Job drawing, mm, ordinate dimensions from the low corner. One solid piece. Give positions to 0.01 mm unless a question says otherwise; leave off trailing zeros. Order: outer loops, then holes, each group sorted by start corner. A loop starts at its lowest first (then second) coordinate and runs counter-clockwise, first axis right, second up.
Item 1: Flat gauge pins, fed straight in: P1, Ø1, axis at x = 21, y = 62.5, coming from the +Z side; P2, Ø12, axis at x = 24.5, z = 135.5, coming from the -Y side. Where does each tip first touch, or does it go through?
Item 2: Band-saw the part on D-D on x = 125. Give the cut face in (y, z), plus the area to 3 significant figures.
Item 3: Band-saw the part on A-A on x = 30. Give the cut face in (y, z), plus the area to 3 significant figures.
Item 4: Two-plate mould, pull along Z, no slides. Class the marked faces 1, 2 and 3: released by +Z, released by -Z, zero draft, split by the parting line, or undercut.
Item 5: Band-saw the part on C-C on y = 46. Give the cut face in (x, z), plus the area to 3 significant figures.
Item 6: Band-saw the part on B-B on z = 170. Give the cut face in (x, y).
Item 7: Wall check: L1, parallel to X at y = 125.5, z = 31; L2, parallel to Y at x = 93.5, z = 170.5; L3, parallel to Z at x = 23.5, y = 138.5. Give the ranges that are in metal, low to high.
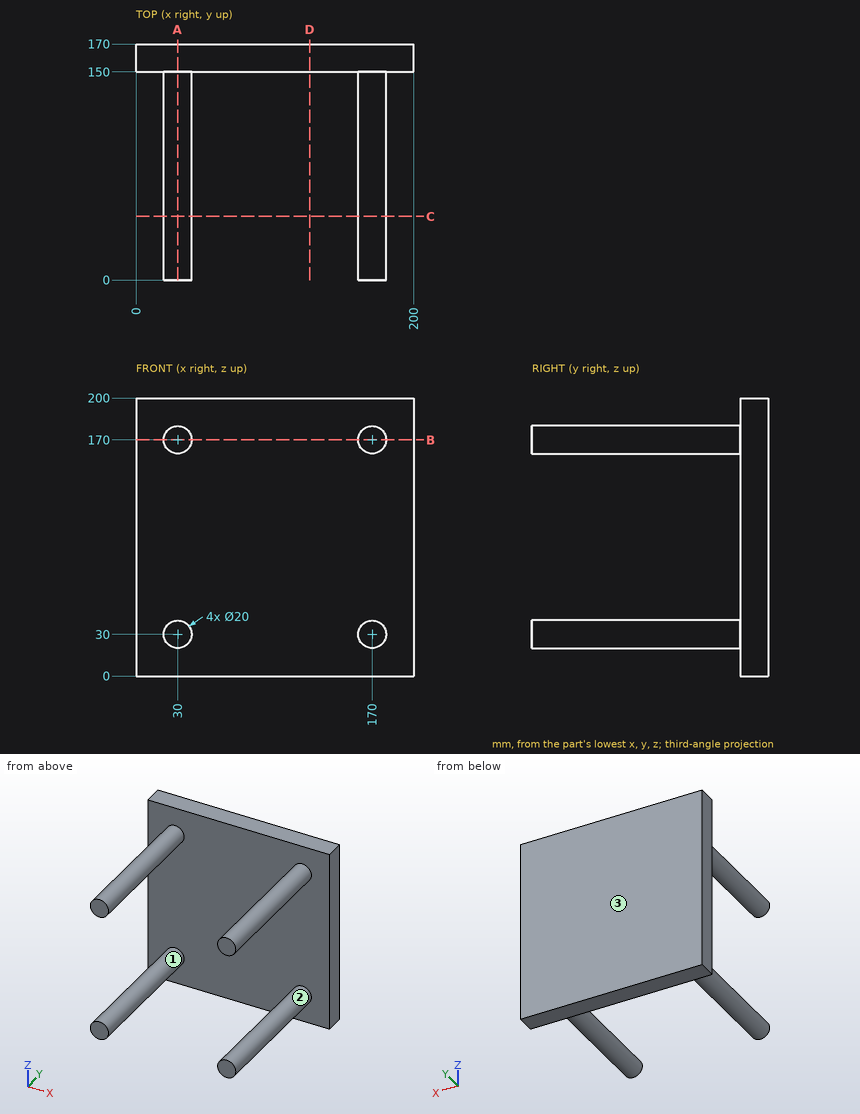
The answers:
1. P1: stops at z = 175.27
1. P2: stops at y = 150
2. outline: (150, 0) - (170, 0) - (170, 200) - (150, 200) - close
2. area: 4,000 mm2
3. outline: (0, 20) - (150, 20) - (150, 0) - (170, 0) - (170, 200) - (150, 200) - (150, 180) - (0, 180) - (0, 160) - (150, 160) - (150, 40) - (0, 40) - close
3. area: 10,000 mm2
4. face 1: undercut
4. face 2: undercut
4. face 3: zero draft
5. outline: circle Ø20 at (30, 30); circle Ø20 at (30, 170); circle Ø20 at (170, 30); circle Ø20 at (170, 170)
5. area: 1,260 mm2
6. outline: (0, 150) - (20, 150) - (20, 0) - (40, 0) - (40, 150) - (160, 150) - (160, 0) - (180, 0) - (180, 150) - (200, 150) - (200, 170) - (0, 170) - close
7. L1: x = 20.05 to 39.95, 160.05 to 179.95
7. L2: y = 150 to 170
7. L3: z = 22.4 to 37.6, 162.4 to 177.6
